Here's how the part is built. I have some questions about the finished solid (model axes, mm). Round coordinates to 2 decimals unless told otherwise and drop trailing zeros. Order: outer loops, then holes, each group sorted by start corner. A loop starts at its lowest first (then second) coordinate and runs counter-clockwise, first axis right, second up. Notation, with made-up numbers: (7, 28.5) -> (38, 28.5) arc R11 ccw to (38, 43.5) -> close; hole circle Ø6 at (0, -0.75). An arc over 180 degrees is marked (long way). One line per item, written item: value.
```python
from build123d import *

# Parameters (mm, degrees)
ESQUISSE1_W                   = 270
ESQUISSE1_H                   = 218
BOSS_EXTRU_1_DEPTH            = 3
ESQUISSE3_R                   = 3
ENL_V_MAT_EXTRU_1_DEPTH       = 10
ESQUISSE4_R                   = 3
ENL_V_MAT_EXTRU_2_DEPTH       = 10
ENL_V_MAT_EXTRU_11_DEPTH      = 174.536739626
ENL_V_MAT_EXTRU_11_DEPTH_BACK = 174.536739626


with BuildPart() as part:
    # Esquisse1 → Boss.-Extru.1 (new body)
    with BuildSketch(Plane.XY):
        Rectangle(ESQUISSE1_W, ESQUISSE1_H)
    extrude(amount=BOSS_EXTRU_1_DEPTH)

    # Esquisse3 → Enlèv. mat.-Extru.1 (cut)
    with BuildSketch(Plane.XY.offset(3)):
        with Locations((-100, -24)):
            Circle(ESQUISSE3_R)
    extrude(amount=-ENL_V_MAT_EXTRU_1_DEPTH, mode=Mode.SUBTRACT)

    # Esquisse4 → Enlèv. mat.-Extru.2 (cut)
    with BuildSketch(Plane.XY.offset(3)):
        with Locations((-75, 55.5)):
            Circle(ESQUISSE4_R)
    extrude(amount=-ENL_V_MAT_EXTRU_2_DEPTH, mode=Mode.SUBTRACT)

    # Esquisse5 → Enlèv. mat.-Extru.11 (cut, two sides: drawn at the far end of the back side and taken through both)
    with BuildSketch(Plane.XY.offset(3).offset(-ENL_V_MAT_EXTRU_11_DEPTH_BACK)):
        Polygon((135, -39), (53.963742643, -46.089753853), (-55, -109), (135, -109), align=None)
    extrude(amount=ENL_V_MAT_EXTRU_11_DEPTH + ENL_V_MAT_EXTRU_11_DEPTH_BACK, mode=Mode.SUBTRACT)


solid = part.part
```
Q1. I want a section at D-D on y = -66. Write out the boundary of the cut face in (x, z).
Answers:
outline: (-135, 0) -> (19.48, 0) -> (19.48, 3) -> (-135, 3) -> close
Q2. I want a section at B-B on x = -100. Write out the boundary of the cut face in (y, z), then the cut area to 3 significant figures.
Answers:
outline: (-109, 0) -> (-27, 0) -> (-27, 3) -> (-109, 3) -> close; (-21, 0) -> (109, 0) -> (109, 3) -> (-21, 3) -> close
area: 636 mm2
Q3. I want a section at C-C on z = 0.9. Write out the boundary of the cut face in (x, y), then the cut area to 3 significant figures.
Answers:
outline: (-135, -109) -> (-55, -109) -> (53.96, -46.09) -> (135, -39) -> (135, 109) -> (-135, 109) -> close; hole circle Ø6 at (-100, -24); hole circle Ø6 at (-75, 55.5)
area: 50,000 mm2
Q4. For P1, Ø5, axis at x = -100, y = -24, coming from the +Z side; P2, Ø8, axis at x = -75, y = 55.5, coming from the -Z side, each with a flat end and sliding along its axis, tell me the tip position at first contact or that it passes through.
Answers:
P1: through
P2: z = 0
Q5. I want a section at A-A on y = 55.5. Write out the boundary of the cut face in (x, z), then the cut area to 3 significant figures.
Answers:
outline: (-135, 0) -> (-78, 0) -> (-78, 3) -> (-135, 3) -> close; (-72, 0) -> (135, 0) -> (135, 3) -> (-72, 3) -> close
area: 792 mm2
Q6. I need wall thicknesses on line 1 along Y through (x, z) = (-75, 1.4); line 2 along Y through (x, z) = (-100, 0.95); line 3 along Y through (x, z) = (27, 2.2). Which ranges of each line are inside material? Lowest first, please.
Answers:
line 1: -109 to 52.5, 58.5 to 109
line 2: -109 to -27, -21 to 109
line 3: -61.66 to 109
Q7. If we mould it in two halves opening along Y, with no side actions, what happens to faces 1 (the face through (-2, 26, 0)), 2 (the face through (0.245, -77.105, 1.479)), 3 (the face through (-103, -24, 2))? For each: pulls with the +Y half, pulls with the -Y half, needs draft (parallel to the pull), parting line crosses it, or undercut.
Answers:
face 1: needs draft
face 2: pulls with the -Y half
face 3: undercut
